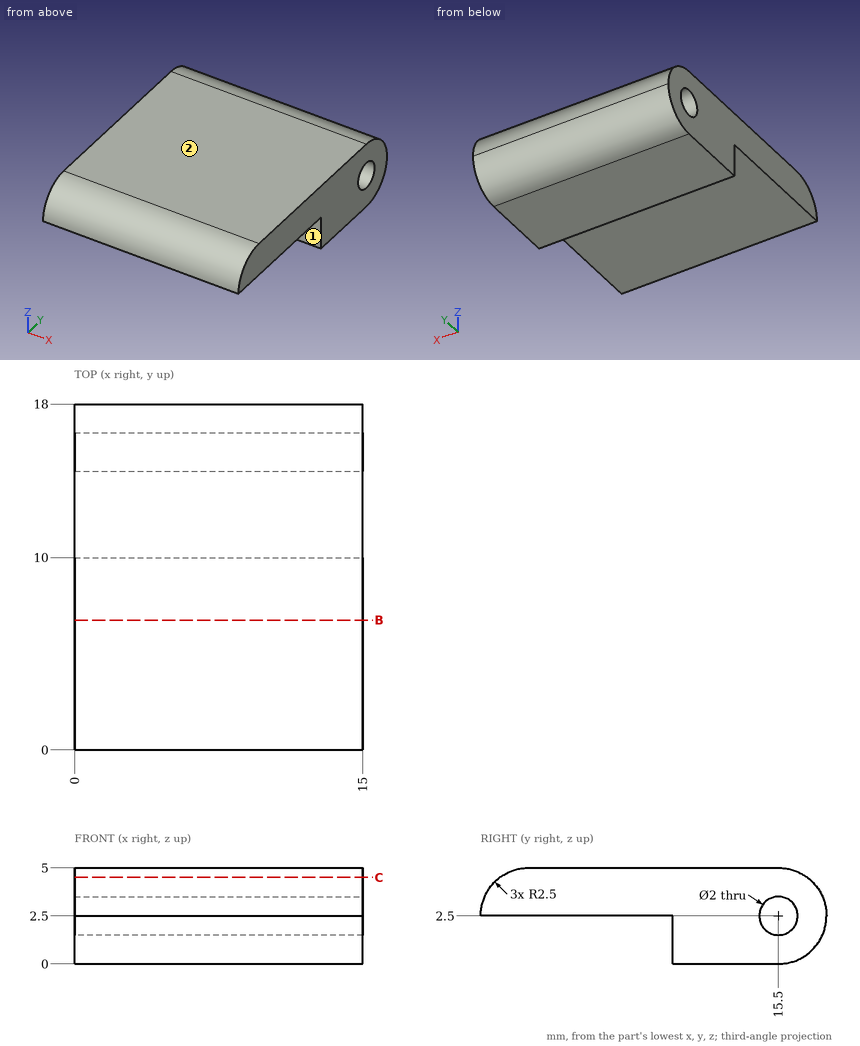
Input: dimensioned drawing with shaded views. Units: mm. Origin: part minimum x, y, z. A direction names the side the tool comes from. Coordinates: 2 decimals unless noted, no trailing zeros. Order: outer loops, then holes, each group sorted by start corner. A loop starts at its lowest first (then second) coordinate and runs counter-clockwise, first axis right, second up.
(1) Material intervals for probe 1 along Y at (x, z) = (4, 2.05); probe 2 along Z at (x, y) = (8.5, 8); probe 3 along Y at (x, z) = (14.25, 4.7), sorted ascending.
(2) First-contact query: pin 1 (1.8 mm diameter, centred on y = 15.5, z = 2.5, fed in from -X); pin 2 (3 mm diameter, centred on x = 8.5, y = 6, fed in from -Z). Flat tips, straight axial feed; report the tip coordinate or a pass-through.
(3) Section query C-C (z = 4.5). Return the cut outline in (x, y), plus the area to 3 significant figures.
(4) Access query for the marked faces 1 and 2. Directions: +Z, -Z, +X, -X, +Y, -Y. A direction counts if a zero-diameter tool reaches every point of the face in a straight line with its end or side. Return the directions, or none.
(5) Section query B-B (y = 6.75). Return the cut outline in (x, z), plus the area to 3 significant figures.
Solution:
1. probe 1: y = 10 to 14.61, 16.39 to 17.96
1. probe 2: z = 2.5 to 5
1. probe 3: y = 1.31 to 16.69
2. pin 1: passes through
2. pin 2: stops at z = 2.5
3. outline: (0, 1) - (15, 1) - (15, 17) - (0, 17) - close
3. area: 240 mm2
4. face 1: -Z, +X, -X, -Y
4. face 2: +Z, +X, -X, +Y, -Y
5. outline: (0, 2.5) - (15, 2.5) - (15, 5) - (0, 5) - close
5. area: 37.5 mm2
